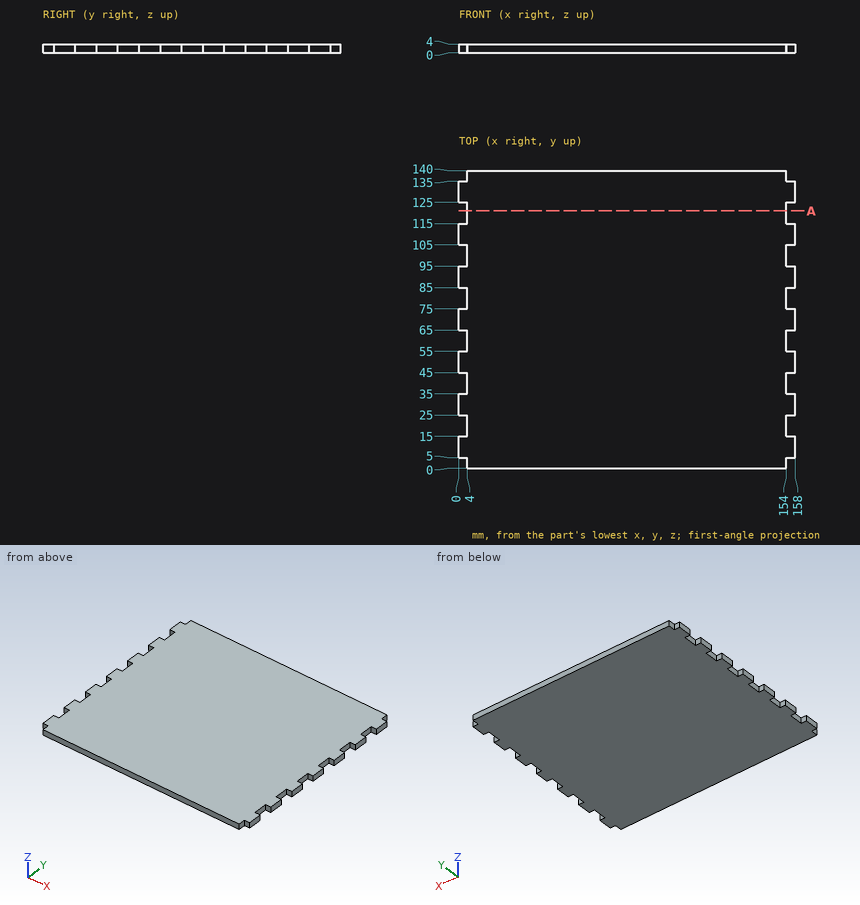
The drawing under review shows one solid part. Ordinate dimensions are in mm from its lowest x, y, z. Round coordinates to 2 decimals unless told otherwise and drop trailing zeros. Order: outer loops, then holes, each group sorted by start corner. A loop starts at its lowest first (then second) coordinate and runs counter-clockwise, first axis right, second up. Notation, with made-up numbers: (-33, 5.25) - (-2, 5.25) arc R8 cw to (-2, 10.25) - close; hole circle Ø5 at (89, 54.5). An arc over 180 degrees is marked (long way). Return JSON: item names as keys, results as strings.
Q1. For pin 1 Ø1 at (y, z) = (18.5, 3.5) entering from +X; pin 2 Ø2 at (y, z) = (118, 2.5) entering from -X; pin 3 Ø1.2 at (x, z) = (2.5, 2) entering from -Y, all flat-tipped, find the tip position at first contact; note any pin that passes through.
Computed values:
{"pin 1": "stops at x = 154", "pin 2": "stops at x = 4", "pin 3": "stops at y = 5"}
Q2. Wall thickness on L1, parallel to X at y = 22, z = 1.65: over which ranges is the line inside the solid? List them lowest first. Write a range as [from, to].
Computed values:
{"L1": "x = [4, 154]"}
Q3. Consider section A-A on y = 121. Write out the cut boundary in (x, z), plus the area to 3 significant figures.
Computed values:
{"outline": "(4, 0) - (154, 0) - (154, 4) - (4, 4) - close", "area": "600 mm2"}
